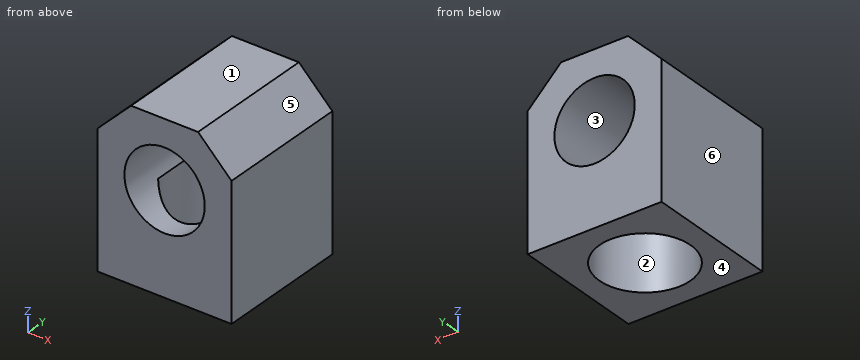
```python
from build123d import *

# Parameters (mm, degrees)
F0_R     = 3
F1_DEPTH = 5
F2_R     = 3.4
F3_DEPTH = 6
F4_SIZE  = 2.5


with BuildPart() as f1:
    # F0 (on Front) → F1 (new body, symmetric)
    with BuildSketch(Plane.XZ):
        Polygon((5, 5), (-5, 5), (-5, -5), (-5, -7.5), (5, -7.5), (5, -5), align=None)
        Circle(F0_R, mode=Mode.SUBTRACT)
    extrude(amount=F1_DEPTH, both=True)

    # F2 (on face) → F3 (cut)
    with BuildSketch(Plane(origin=(0, 0, -7.5), x_dir=(1, 0, 0), z_dir=(0, 0, -1))):
        Circle(F2_R)
    extrude(amount=-F3_DEPTH, mode=Mode.SUBTRACT)

    # F4
    f4_edges = [f1.edges().sort_by_distance(p)[0] for p in [
        (-5, 0, 5),
        (5, 0, 5),
    ]]
    chamfer(f4_edges, length=F4_SIZE)


solid = f1.part
```
The listing builds one solid part. Answer for the finished solid, in the listing's coordinates (mm). Face numbers are marked on the shaded views. A direction names the side the tool comes from. Round coordinates to 2 decimals unless told otherwise and drop trailing zeros. Order: outer loops, then holes, each group sorted by start corner. A loop starts at its lowest first (then second) coordinate and runs counter-clockwise, first axis right, second up. Notation, with made-up numbers: (68, 39) - (85, 39) arc R36 ccw to (85, 77) - close; hole circle Ø4 at (19.5, 73). An arc over 180 degrees is marked (long way). Put each result on its own line as item: value. Start each with the question number.
(1) Find section B-B (y = -3.75). Give the vertices of the cut face in (x, z), plus the area to 3 significant figures.
(2) Given P1, Ø0.6, axis at x = -3, y = 0, coming from the -Z side; P2, Ø2, axis at x = 2.5, z = -0.5, coming from the -Y side, each flat-ended and moving along its own axis, determine where each tip first touches the part or whether it passes through.
(3) For the marked faces 1 and 2, determine the directions among +Z, -Z, +X, -X, +Y, -Y from which every point of the face is accessible in a straight line to the end or side of a thin tool.
(4) Find section D-D (y = 0). Give the vertices of the cut face in (x, z), plus the area to 3 significant figures.
(5) Find section A-A (x = 0). Give the vertices of the cut face in (y, z), plus the area to 3 significant figures.
(6) Determine the mould class of the marked faces 3, 4, 5 and 6 for opening direction X: released by +X, released by -X, zero draft, split by the parting line, or undercut.
(7) Straight lines are drawn through the part: probe 1 along Y at (x, z) = (0, -3.5); probe 2 along Z at (x, y) = (-1.5, -2.5). For each, find the intervals that lie inside material, in ascending order. Write a range as from..to.
(8) Find section C-C (z = 0). Give the vertices of the cut face in (x, y).
Reply:
1. outline: (-5, -7.5) - (5, -7.5) - (5, 2.5) - (2.5, 5) - (-2.5, 5) - (-5, 2.5) - close; hole circle Ø6 at (0, 0)
1. area: 90.5 mm^2
2. P1: z = -1.5
2. P2: y = -5
3. face 1: +Z, +X, -X, +Y, -Y
3. face 2: -Z
4. outline: (-5, -7.5) - (-3.4, -7.5) - (-3.4, -1.5) - (-2.6, -1.5) arc R3 cw (long way) to (2.6, -1.5) - (3.4, -1.5) - (3.4, -7.5) - (5, -7.5) - (5, 2.5) - (2.5, 5) - (-2.5, 5) - (-5, 2.5) - close
4. area: 55.2 mm^2
5. outline: (-5, -7.5) - (-3.4, -7.5) - (-3.4, -3) - (-5, -3) - close; (-5, 3) - (5, 3) - (5, 5) - (-5, 5) - close; (3.4, -7.5) - (5, -7.5) - (5, -3) - (3.4, -3) - close
5. area: 34.4 mm^2
6. face 3: undercut
6. face 4: zero draft
6. face 5: released by +X
6. face 6: released by -X
7. probe 1: -5..-3.4, 3.4..5
7. probe 2: 2.6..5
8. outline: (-5, -5) - (-3, -5) - (-3, 5) - (-5, 5) - close; (3, -5) - (5, -5) - (5, 5) - (3, 5) - close
